Verification items for this drawing (mm, ordinates from the low corner). Round coordinates to 2 decimals unless told otherwise and drop trailing zeros. Order: outer loops, then holes, each group sorted by start corner. A loop starts at its lowest first (then second) coordinate and runs counter-clockwise, first axis right, second up. Notation, with made-up numbers: (15, 44) -> (25, 44) arc R27 cw to (25, 61) -> close; hole circle Ø4 at (50, -6.75). An arc over 180 degrees is marked (long way). Return JSON: item names as keys, results as strings. Group by question number.
Item 1: Sectioned sample at A-A on z = 30.5. Record the cut outline in (x, y) (1 decimal).
Item 2: Scan lines: probe 1 along Z at (x, y) = (8.5, 1.35) (1 decimal); probe 2 along Z at (x, y) = (43.5, 0.7) (1 decimal); probe 3 along X at (y, z) = (1.1, 39) (1 decimal). Record each from-to range of solid material in increasing order. Write a range as from..to.
Item 3: Sectioned sample at B-B on x = 44.45. Record the cut outline in (y, z) (1 decimal), plus the area to 3 significant figures.
Item 4: Depth check by flat-ended pin: pin 1 Ø4 at (x, z) = (44.45, 85.725) entering from -Y. Enter the tip coordinate at first touch or a pass-through.
Item 5: Sectioned sample at D-D on z = 44.45. Record the cut outline in (x, y), plus the area to 3 significant figures.
Item 6: Sectioned sample at C-C on y = 1.55. Give the number of separate pieces and of enclosed holes in the cut face, plus the area to 3 significant figures.
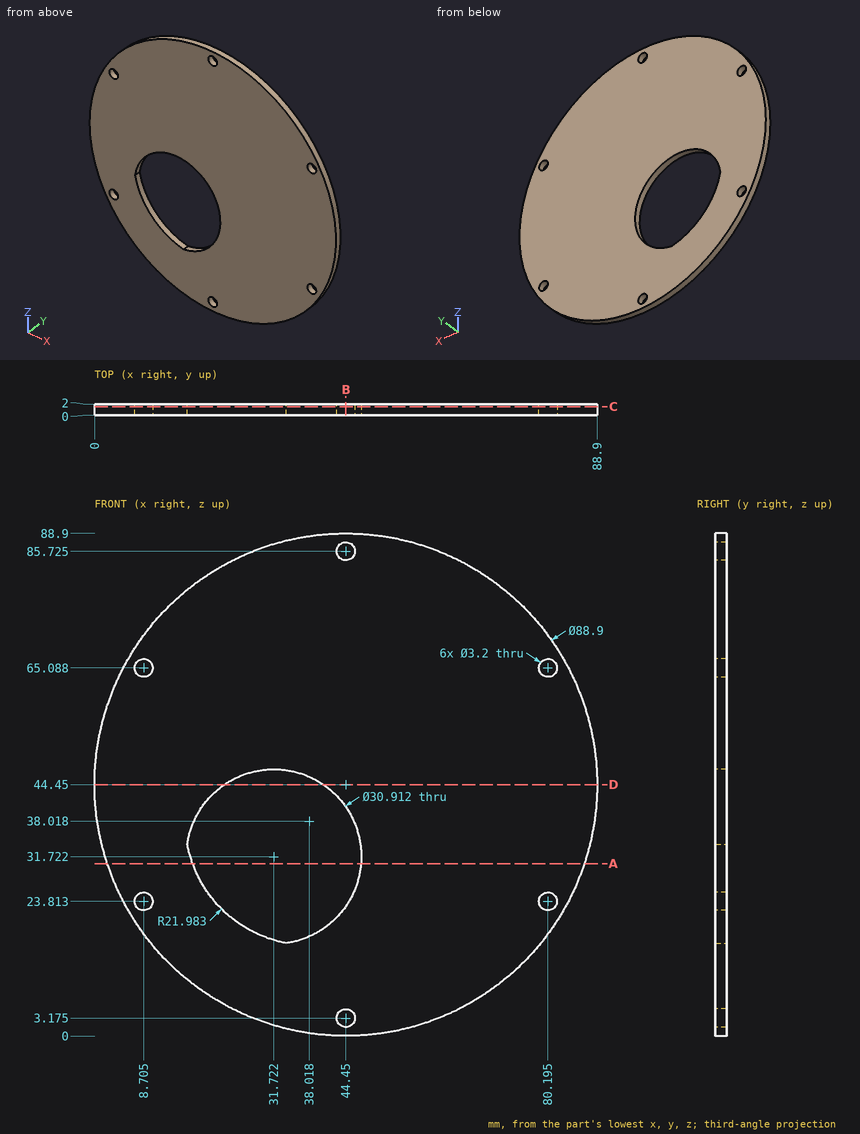
Recorded:
{
 "1": {"outline": "(2.2, 0) -> (17.4, 0) -> (17.4, 2) -> (2.2, 2) -> close; (47.1, 0) -> (86.7, 0) -> (86.7, 2) -> (47.1, 2) -> close"},
 "2": {"probe 1": "18.3..22.2, 25.4..63.5, 66.7..70.6", "probe 2": "0..1.9, 4.5..21.7, 41.7..84.4, 87..88.9", "probe 3": "0.3..18.1, 45.4..88.6"},
 "3": {"outline": "(0, 0) -> (2, 0) -> (2, 1.6) -> (0, 1.6) -> close; (0, 4.8) -> (2, 4.8) -> (2, 23) -> (0, 23) -> close; (0, 40.5) -> (2, 40.5) -> (2, 84.1) -> (0, 84.1) -> close; (0, 87.3) -> (2, 87.3) -> (2, 88.9) -> (0, 88.9) -> close", "area": "130 mm²"},
 "4": {"pin 1": "y = 0"},
 "5": {"outline": "(0, 0) -> (22.95, 0) -> (22.95, 2) -> (0, 2) -> close; (40.49, 0) -> (88.9, 0) -> (88.9, 2) -> (40.49, 2) -> close", "area": "143 mm²"},
 "6": {"separate pieces": "1", "enclosed holes": "7", "area": "5,450 mm²"}
}
